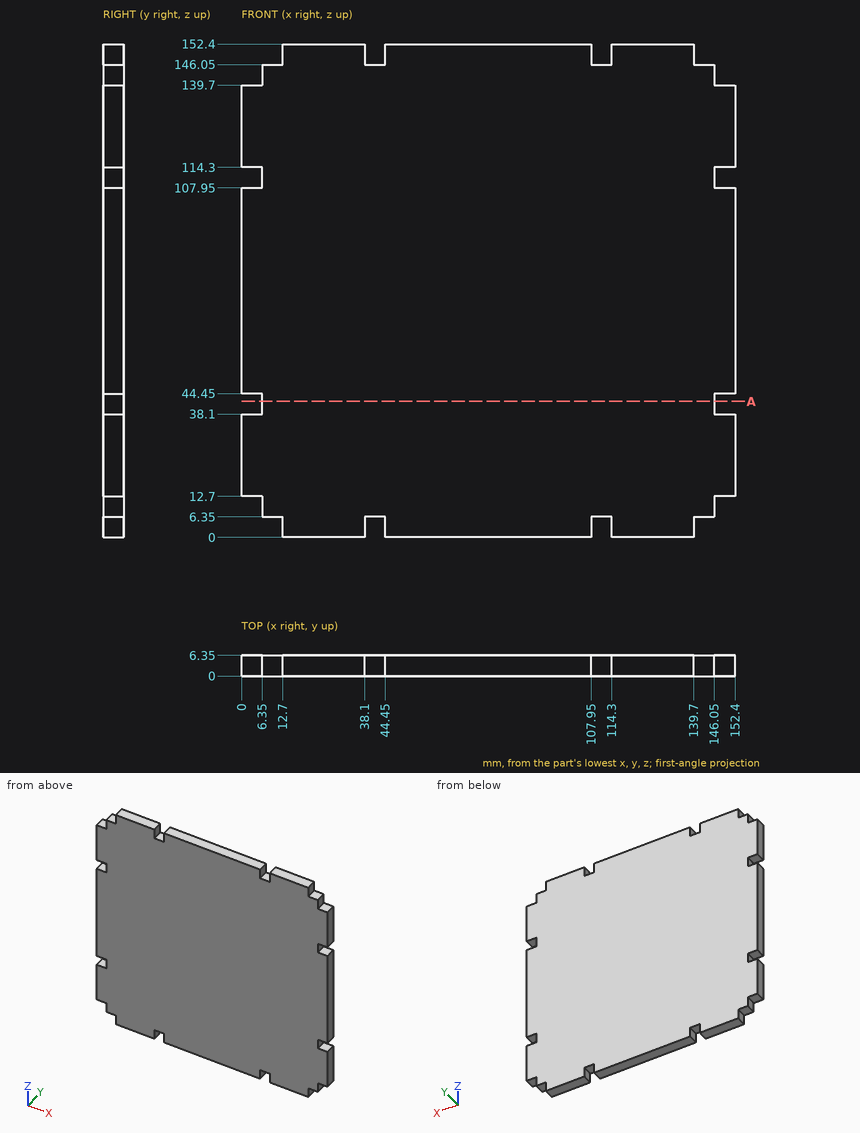
Geometry check sheet. Reference: drawing and pictorial views, mm from the part's lowest x, y, z. Coordinates: 2 decimals unless noted, no trailing zeros. Order: outer loops, then holes, each group sorted by start corner. A loop starts at its lowest first (then second) coordinate and runs counter-clockwise, first axis right, second up.
Item 1: Depth check by flat-ended pin: pin 1 (1.9 mm diameter, centred on x = 3, y = 2.5, fed in from +Z); pin 2 (1.9 mm diameter, centred on x = 4.5, y = 3, fed in from -Z); pin 3 (3 mm diameter, centred on y = 3, z = 2.5, fed in from +X). Enter the tip coordinate at first touch or a pass-through.
Item 2: Scan line: line 1 along X through (y, z) = (1.75, 113). Record every from-to range of solid material in increasing order.
Item 3: Section check A-A (z = 42). Enter the section's corners in (x, y).
Check sheet entries:
1. pin 1: stops at z = 139.7
1. pin 2: stops at z = 12.7
1. pin 3: stops at x = 139.7
2. line 1: x = 6.35 to 146.05
3. outline: (6.35, 0) - (146.05, 0) - (146.05, 6.35) - (6.35, 6.35) - close
